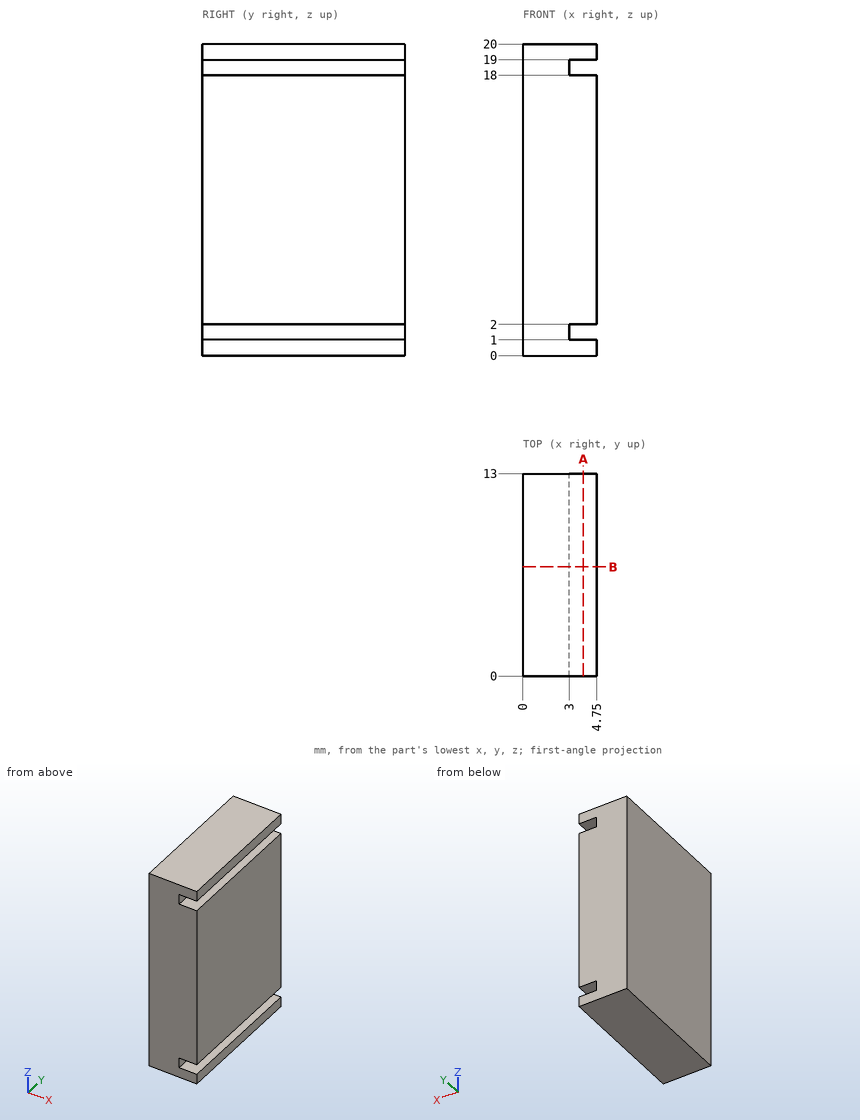
Check sheet for the drawn part. Datum: minimum x, y, z corner. Units: mm. Round coordinates to 2 decimals unless told otherwise and drop trailing zeros. Loops run counter-clockwise (first coordinate to the right, second up) from the corner with the lowest first, then second, coordinate; pieces in that order, holes last. Notation, with made-up numbers: (-6, -0.5) - (24, -0.5) arc R9 cw to (24, 11.5) - close; hole circle Ø9 at (75, -9). An arc over 180 degrees is marked (long way). Write item = value, one per line. Start each with the question number.
1. Section check B-B on y = 7. Enter the section's corners in (x, z).
2. Thickness scan on line 1 (Z direction, x = 3.9, y = 10.5); line 2 (X direction, y = 4.75, z = 18.75). Record the ranges inside material, lowest first.
3. Section check A-A on x = 3.9. Enter the section's corners in (y, z).
4. Depth check by flat-ended pin: pin 1 (3 mm diameter, centred on y = 11, z = 2, fed in from -X); pin 2 (0.5 mm diameter, centred on y = 6, z = 18.5, fed in from +X). Enter the tip coordinate at first touch or a pass-through.
Working result:
q1.outline = (0, 0) - (4.75, 0) - (4.75, 1) - (3, 1) - (3, 2) - (4.75, 2) - (4.75, 18) - (3, 18) - (3, 19) - (4.75, 19) - (4.75, 20) - (0, 20) - close
q2.line_1 = 0 to 1, 2 to 18, 19 to 20
q2.line_2 = 0 to 3
q3.outline = (0, 0) - (13, 0) - (13, 1) - (0, 1) - close; (0, 2) - (13, 2) - (13, 18) - (0, 18) - close; (0, 19) - (13, 19) - (13, 20) - (0, 20) - close
q4.pin_1 = 0
q4.pin_2 = 3
